```python
from build123d import *

# Parameters (mm, degrees)
SKETCH_1_W      = 11.35
SKETCH_1_H      = 5.65
SKETCH_1_W_2    = 10.35
SKETCH_1_H_2    = 4.65
EXTRUDE_1_DEPTH = 9.5
SCALE_1_SCALE   = 1.2


with BuildPart() as part:
    # 草图1 → 拉伸-薄壁1 (new body)
    with BuildSketch(Plane.XY):
        Rectangle(SKETCH_1_W, SKETCH_1_H)
        Rectangle(SKETCH_1_W_2, SKETCH_1_H_2, mode=Mode.SUBTRACT)
    extrude(amount=EXTRUDE_1_DEPTH)


with BuildPart() as part_1:
    # 缩放比例1: scaled about (0, 0, 4.75)
    add(part.part.scale(SCALE_1_SCALE).moved(Location((0, 0, -0.95))))


solid = part_1.part
```
For this review, take the finished solid that the model builds, in its own axes (mm). A direction names the side the tool comes from. Round coordinates to 2 decimals unless told otherwise and drop trailing zeros. Write each loop counter-clockwise with the first axis right and the second up, starting at its lowest first coordinate (ties: lowest second). Pieces come first, ordered by that corner, then holes. Notation, with made-up numbers: (72.25, -1.5) -> (118.25, -1.5) arc R15 ccw to (118.25, 4.5) -> close; hole circle Ø5 at (53, 16). An arc over 180 degrees is marked (long way). Use one line per item in the form item = value.
Q1. Consider section C-C (x = 5.5). State the section outline as (y, z) points, then the cut area to 3 significant figures.
Resolved:
outline = (-3.39, -0.95) -> (-2.79, -0.95) -> (-2.79, 10.45) -> (-3.39, 10.45) -> close; (2.79, -0.95) -> (3.39, -0.95) -> (3.39, 10.45) -> (2.79, 10.45) -> close
area = 13.7 mm²
Q2. Consider section B-B (y = 1.25). State the section outline as (x, z) points.
Resolved:
outline = (-6.81, -0.95) -> (-6.21, -0.95) -> (-6.21, 10.45) -> (-6.81, 10.45) -> close; (6.21, -0.95) -> (6.81, -0.95) -> (6.81, 10.45) -> (6.21, 10.45) -> close
Q3. Machinability: for faces 4 (the flat face through (6.21, 0, 5)), 5 (the flat face through (0, 3.39, 5)), which of the approach directions +Z, -Z, +X, -X, +Y, -Y give a long, thin tool a straight path to every point of the face, cutting with its end or side? Answer none if there is none.
Resolved:
face_4 = +Z, -Z
face_5 = +Z, -Z, +X, -X, +Y
Q4. The part is to be moulded in two halves that separate along Y. For faces 1 (the flat face through (0, -3.39, 5)), 2 (the flat face through (6.81, 0, 5)), 3 (the flat face through (0, -2.79, 5)), say which applies: released by +Y, released by -Y, zero draft, split by the parting line, or undercut.
Resolved:
face_1 = released by -Y
face_2 = zero draft
face_3 = undercut
Q5. To check wall thickness, follow probe 1 along X at (y, z) = (-2.5, 10.25); probe 2 along Y at (x, z) = (-5.25, 0). State the ranges of each line that lie inside material, in increasing order. Write a range as from..to.
Resolved:
probe_1 = -6.81..-6.21, 6.21..6.81
probe_2 = -3.39..-2.79, 2.79..3.39
Q6. Consider section A-A (z = 1.5). State the section outline as (x, y) points, then the cut area to 3 significant figures.
Resolved:
outline = (-6.81, -3.39) -> (6.81, -3.39) -> (6.81, 3.39) -> (-6.81, 3.39) -> close; hole (-6.21, -2.79) -> (6.21, -2.79) -> (6.21, 2.79) -> (-6.21, 2.79) -> close
area = 23.0 mm²
Q7. Clearance check with a flat-ended pin moving along its axis: pin 1 Ø1.5 at (x, y) = (1.5, 0.5) entering from +Z. State where the tip first meets the part, or that it passes through.
Resolved:
pin_1 = through
